from build123d import *

# Parameters (mm, degrees)
SKETCH1_W           = 100
SKETCH1_H           = 45
SKETCH1_R           = 4
SKETCH1_R_2         = 3.6
BOSS_EXTRUDE1_DEPTH = 25
SKETCH1_3_R         = 11
CUT_EXTRUDE1_DEPTH  = 7.5
FILLET1_R           = 5
SKETCH1_4_R         = 7
CUT_EXTRUDE2_DEPTH  = 8


with BuildPart() as part:
    # Sketch1 → Boss-Extrude1 (new body)
    with BuildSketch(Plane.XY):
        with Locations((50, 22.5)):
            Rectangle(SKETCH1_W, SKETCH1_H)
        with Locations((20, 12.5)):
            Circle(SKETCH1_R, mode=Mode.SUBTRACT)
        with Locations((50, 32)):
            Circle(SKETCH1_R_2, mode=Mode.SUBTRACT)
        with Locations((80, 12.5)):
            Circle(SKETCH1_R, mode=Mode.SUBTRACT)
    extrude(amount=BOSS_EXTRUDE1_DEPTH)

    # Sketch1<3> → Cut-Extrude1 (cut)
    with BuildSketch(Plane.XY):
        with Locations((50, 32)):
            Circle(SKETCH1_3_R)
    extrude(amount=CUT_EXTRUDE1_DEPTH, mode=Mode.SUBTRACT)

    # Fillet1
    fillet1_edges = [part.edges().sort_by_distance(p)[0] for p in [
        (100, 45, 12.5),
        (0, 45, 12.5),
    ]]
    fillet(fillet1_edges, radius=FILLET1_R)

    # Sketch1<4> → Cut-Extrude2 (cut)
    with BuildSketch(Plane.XY):
        with Locations((80, 12.5)):
            Circle(SKETCH1_4_R)
        with Locations((20, 12.5)):
            Circle(SKETCH1_4_R)
    extrude(amount=CUT_EXTRUDE2_DEPTH, mode=Mode.SUBTRACT)


solid = part.part
CAD build for the part. Positions are in the model's coordinates, mm. A direction names the side the tool comes from. Round coordinates to 2 decimals unless told otherwise and drop trailing zeros. Write each loop counter-clockwise with the first axis right and the second up, starting at its lowest first coordinate (ties: lowest second). Pieces come first, ordered by that corner, then holes. Notation, with made-up numbers: (80.25, -34.5) -> (111.25, -34.5) arc R23 ccw to (111.25, 1.5) -> close; hole circle Ø9 at (58, 19.5). An arc over 180 degrees is marked (long way). Answer as a JSON object with one key per item and string values.
(1) Probe probe 1 along X at (y, z) = (12.5, 12); probe 2 along Y at (x, z) = (50.5, 2); probe 3 along X at (y, z) = (11, 7.5). List the from-to ranges inside material, lowest first. Write a range as [from, to].
Reported:
{"probe 1": "x = [0, 16], [24, 76], [84, 100]", "probe 2": "y = [0, 21.01], [42.99, 45]", "probe 3": "x = [0, 13.16], [26.84, 73.16], [86.84, 100]"}
(2) Two-plate mould, pull along X, no slides. Class faces 1 (the face through (23, 9, 8)), 2 (the face through (1, 43, 13)), 3 (the face through (49, 18, 0)): +X half, -X half, draft (parallel to the pull), parting line (faces both ways), or undercut.
Reported:
{"face 1": "undercut", "face 2": "-X half", "face 3": "draft"}
(3) Pin check, flat tips, straight feed: P1, Ø7, axis at x = 78.5, y = 13.5, coming from the -Z side; P2, Ø5, axis at x = 20, y = 12.5, coming from the -Z side; P3, Ø9.5, axis at x = 50, y = 32, coming from the -Z side. Stop position of each tip, or through.
Reported:
{"P1": "stops at z = 8", "P2": "passes through", "P3": "stops at z = 7.5"}
(4) Which spindle directions (+Z, -Z, +X, -X, +Y, -Y) get a long thin tool onto all of the face, cutting with end or side? Do faces 4 (the face through (51.935, 35.036, 16.127)), 5 (the face through (60.161, 27.787, 3.698)). Say none if no direction does.
Reported:
{"face 4": "+Z, -Z", "face 5": "-Z"}
(5) Band-saw the part on D-D, the plane y = 12.5. List the corners of the cut face in (x, z), then the cut area to 3 significant figures.
Reported:
{"outline": "(0, 0) -> (13, 0) -> (13, 8) -> (16, 8) -> (16, 25) -> (0, 25) -> close; (24, 8) -> (27, 8) -> (27, 0) -> (73, 0) -> (73, 8) -> (76, 8) -> (76, 25) -> (24, 25) -> close; (84, 8) -> (87, 8) -> (87, 0) -> (100, 0) -> (100, 25) -> (84, 25) -> close", "area": "2,000 mm^2"}
(6) Band-saw the part on A-A, the plane y = 32. List the corners of the cut face in (x, z), then the cut area to 3 significant figures.
Reported:
{"outline": "(0, 0) -> (39, 0) -> (39, 7.5) -> (46.4, 7.5) -> (46.4, 25) -> (0, 25) -> close; (53.6, 7.5) -> (61, 7.5) -> (61, 0) -> (100, 0) -> (100, 25) -> (53.6, 25) -> close", "area": "2,210 mm^2"}
(7) Band-saw the part on C-C, the plane z = 21. List the corners of the cut face in (x, y), then the cut area to 3 significant figures.
Reported:
{"outline": "(0, 0) -> (100, 0) -> (100, 40) arc R5 ccw to (95, 45) -> (5, 45) arc R5 ccw to (0, 40) -> close; hole circle Ø8 at (20, 12.5); hole circle Ø7.2 at (50, 32); hole circle Ø8 at (80, 12.5)", "area": "4,350 mm^2"}
(8) Band-saw the part on B-B, the plane x = 20. List the corners of the cut face in (y, z).
Reported:
{"outline": "(0, 0) -> (5.5, 0) -> (5.5, 8) -> (8.5, 8) -> (8.5, 25) -> (0, 25) -> close; (16.5, 8) -> (19.5, 8) -> (19.5, 0) -> (45, 0) -> (45, 25) -> (16.5, 25) -> close"}
